```python
from build123d import *

# Parameters (mm, degrees)
F3_DEPTH = 25
F5_DEPTH = 12.5


# Not quite as in the source:
# - a feature of the source that left no trace in its solid (it failed there, or was rolled back) is left out


with BuildPart() as f1:
    # F0 (on Right) → F1 (revolve)
    with BuildSketch(Plane.YZ):
        Polygon((-1, 2), (0, 2), (1, 2), (1, 3.5723834783), (25, 3.7818283052), (25, 5.7818283052), (0, 6), (-25, 5.7818283052), (-25, 3.7818283052), (-1, 3.5723834783), align=None)
    revolve(axis=Axis((0, 180.1521787086, 0), (0, 1, 0)))

    # F2 (on Top) → F3 (cut)
    with BuildSketch(Plane.XY):
        with BuildLine():
            Line((-3.2170944919, 24.0348994967), (-2.5, 3.5))
            ThreePointArc((-2.5, 3.5), (0, 1), (2.5, 3.5))
            Line((2.5, 3.5), (3.2170944919, 24.0348994967))
            ThreePointArc((3.2170944919, 24.0348994967), (3.5218269484, 24.7193398003), (4.2164853189, 25))
            Line((4.2164853189, 25), (5.7818283052, 25))
            Line((5.7818283052, 25), (5.7818283052, 27.9599502683))
            Line((5.7818283052, 27.9599502683), (-5.9923287481, 27.9599502683))
            Line((-5.9923287481, 27.9599502683), (-5.7818283052, 25))
            Line((-5.7818283052, 25), (-4.2164853189, 25))
            ThreePointArc((-4.2164853189, 25), (-3.5218269484, 24.7193398003), (-3.2170944919, 24.0348994967))
        make_face()
    extrude(amount=F3_DEPTH, mode=Mode.SUBTRACT)

    # F4 (on Right) → F5 (cut, symmetric)
    with BuildSketch(Plane.YZ):
        Polygon((32.3949936356, 6.6679690088), (27.2697879307, 6.7125111288), (9.7397706777, -8.7493574537), (32.3949936356, -8.9470665892), align=None)
        Polygon((-29.6528312787, -5.7412236618), (-25, -5.7818283052), (-3.2005671173, 13.4457606663), (-29.6528312787, 14.9152847007), align=None)
    extrude(amount=F5_DEPTH, both=True, mode=Mode.SUBTRACT)


solid = f1.part
```
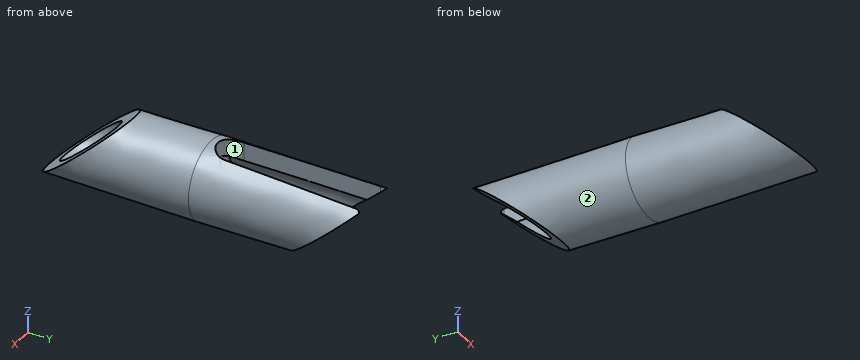
Model file for the job. Use its own axes, mm. Face numbers are marked on the shaded views. Round coordinates to 2 decimals unless told otherwise and drop trailing zeros. Write each loop counter-clockwise with the first axis right and the second up, starting at its lowest first coordinate (ties: lowest second). Pieces come first, ordered by that corner, then holes. Notation, with made-up numbers: (24, 3.25) - (45, 3.25) arc R16 cw to (45, 8.25) - close; hole circle Ø11 at (-23, -22). An arc over 180 degrees is marked (long way). Use CSV: the item, a comma, the result in double quotes. Start each with the question number.
Item 1: Band-saw the part on A-A (y = 14). Write the cut outline in (x, z).
Item 2: Drill centre lines: L1, parallel to X at y = 0.15, z = 0; L2, parallel to X at y = -18.5, z = -0.25; L3, parallel to Z at x = -2.75, y = -10.5. Where is each one in solid material? Low to high. Write a range as [from, to].
Item 3: Band-saw the part on D-D (y = -19.5). Write the cut outline in (x, z).
Item 4: Pin check, flat tips, straight feed: P1, Ø4, axis at x = -2.5, z = -3, coming from the +Y side; P2, Ø4, axis at x = 3.5, z = -3, coming from the +Y side; P3, Ø4.5, axis at x = 0, z = 0, coming from the -Y side. Stop position of each tip, or through.
Item 5: Band-saw the part on C-C (y = -10.5). Write the cut outline in (x, z), and give its area (3 significant figures).
Item 6: Band-saw the part on B-B (y = -5.5). Write the cut outline in (x, z), and give its area (3 significant figures).
Item 7: Two-plate mould, pull along X, no slides. Class the marked faces 1 and 2: released by +X, released by -X, zero draft, split by the parting line, or undercut.
Checked values:
1,outline,"(-3.1, -4.99) - (3.1, -4.99) arc R5.88 ccw to (2.87, 5.13) - (2.87, 2.32) arc R3.69 cw (long way) to (-2.87, 2.32) - (-2.87, 5.13) arc R5.88 ccw to start"
2,L1,"x = [-6, -2], [2, 6]"
2,L2,"x = [-5.83, -3.72], [3.72, 5.83]"
2,L3,"z = [-5.23, -2.41], [2.41, 5.23]"
3,outline,"(-5.76, -0.93) arc R5.83 ccw to (5.76, -0.93) - (3.62, -0.93) arc R3.73 cw to (-3.62, -0.93) - close"
4,P1,"stops at y = 18.22"
4,P2,"stops at y = 18.52"
4,P3,"stops at y = -1"
5,outline,"circle Ø11.82 at (0, 0); hole circle Ø7.31 at (0, 0)"
5,area,"67.7 mm²"
6,outline,"circle Ø11.9 at (0, 0); hole circle Ø7.22 at (0, 0)"
6,area,"70.3 mm²"
7,face 1,"undercut"
7,face 2,"split by the parting line"
